```python
from build123d import *

# Parameters (mm, degrees)
CROQUIS1_R              = 2.5
CROQUIS1_R_2            = 1.6
CROQUIS1_R_3            = 12.5
SALIENTE_EXTRUIR1_DEPTH = 5
REDONDEO1_R             = 5


with BuildPart() as part:
    # Croquis1 → Saliente-Extruir1 (new body)
    with BuildSketch(Plane(origin=(0, 0, 0), x_dir=(1, 0, 0), z_dir=(0, 1, 0))):
        Polygon((51.292156122, 108.840620434), (119.90482032, -10), (46.188021535, -10), (14.43375673, 45), align=None)
        with Locations(Location((51.292156122, 88.840620434, 0), (0, 0, 270))):
            Circle(CROQUIS1_R, mode=Mode.SUBTRACT)
        with Locations(Location((102.584312245, 0, 0), (0, 0, 270))):
            Circle(CROQUIS1_R, mode=Mode.SUBTRACT)
        with Locations(Location((51.961524227, 0, 0), (0, 0, 270))):
            Circle(CROQUIS1_R, mode=Mode.SUBTRACT)
        with Locations(Location((25.980762114, 45, 0), (0, 0, 270))):
            Circle(CROQUIS1_R, mode=Mode.SUBTRACT)
        with Locations(Location((38.97114317, 22.5, 0), (0, 0, 270))):
            Circle(CROQUIS1_R_2, mode=Mode.SUBTRACT)
        with Locations(Location((46.994533568, 52.443700615, 0), (0, 0, 270))):
            Circle(CROQUIS1_R_2, mode=Mode.SUBTRACT)
        with Locations(Location((76.938234183, 44.420310217, 0), (0, 0, 270))):
            Circle(CROQUIS1_R_2, mode=Mode.SUBTRACT)
        with Locations(Location((68.914843785, 14.476609602, 0), (0, 0, 270))):
            Circle(CROQUIS1_R_2, mode=Mode.SUBTRACT)
        with Locations(Location((57.954688677, 33.460155108, 0), (0, 0, 270))):
            Circle(CROQUIS1_R_3, mode=Mode.SUBTRACT)
    extrude(amount=SALIENTE_EXTRUIR1_DEPTH)

    # Redondeo1
    redondeo1_edges = [part.edges().sort_by_distance(p)[0] for p in [
        (51.292156122, 2.5, -108.840620434),
        (119.90482032, 2.5, 10),
        (46.188021535, 2.5, 10),
        (14.43375673, 2.5, -45),
    ]]
    fillet(redondeo1_edges, radius=REDONDEO1_R)


solid = part.part
```
Verification items for the finished model (mm, model axes). Coordinates: 2 decimals unless noted, no trailing zeros. Write each loop counter-clockwise with the first axis right and the second up, starting at its lowest first coordinate (ties: lowest second). Pieces come first, ordered by that corner, then holes. Notation, with made-up numbers: (51, -1) - (109, -1) arc R8 cw to (109, 7) - close; hole circle Ø8 at (1, -23). An arc over 180 degrees is marked (long way). One line per question, with ' | ' between items. Start each with the question number.
1. Section check C-C (z = -22.5). Enter the section's corners in (x, y).
2. Section check A-A (x = 66). Enter the section's corners in (y, z).
3. Section check D-D (z = 0). Enter the section's corners in (x, y).
4. Material ranges on line 1 along Z through (x, y) = (68, 0.5); line 2 along Z through (x, y) = (68.5, 2.4); line 3 along X through (y, z) = (1.7, -22.5), recorded low to high.
5. Section check B-B (y = 2.95). Count the separate pieces of the cut face and the enclosed holes in it, plus the area to 3 significant figures.
6. Gauge pin test, flat ends, axial feed: P1, Ø1.5, axis at y = 1.5, z = -84.5, coming from the -X side; P2, Ø2, axis at x = 61.5, y = 4.5, coming from the -Z side; P3, Ø1.5, axis at x = 31.5, y = 1, coming from the +Z side. Record the tip position at first contact, or that the pin passes through.
7. Draft check along X on faces 1 (the cylindrical face through (46.61, 2.54, 9.35)), 2 (the flat face through (85.179, 2.465, -50.147)), 3 (the cylindrical face through (100.144, 2.465, -0.542)). Enter one of: released by +X, released by -X, zero draft, split by the parting line, or undercut.
Computed values:
1) outline: (27.42, 0) - (37.37, 0) - (37.37, 5) - (27.42, 5) - close; (40.57, 0) - (51.94, 0) - (51.94, 5) - (40.57, 5) - close; (63.97, 0) - (101.14, 0) - (101.14, 5) - (63.97, 5) - close
2) outline: (0, -83.37) - (5, -83.37) - (5, -43.03) - (0, -43.03) - close; (0, -23.89) - (5, -23.89) - (5, 10) - (0, 10) - close
3) outline: (40.41, 0) - (49.46, 0) - (49.46, 5) - (40.41, 5) - close; (54.46, 0) - (100.08, 0) - (100.08, 5) - (54.46, 5) - close; (105.08, 0) - (114.13, 0) - (114.13, 5) - (105.08, 5) - close
4) line 1: -79.9 to -40.9, -26.02 to -15.79, -13.16 to 10 | line 2: -79.04 to -40.17, -26.75 to -16.02, -12.93 to 10 | line 3: 27.42 to 37.37, 40.57 to 51.94, 63.97 to 101.14
5) separate pieces: 1 | enclosed holes: 9 | area: 5,770 mm²
6) P1: x = 36.81 | P2: z = -92.89 | P3: z = -14.14
7) face 1: released by -X | face 2: released by +X | face 3: undercut
